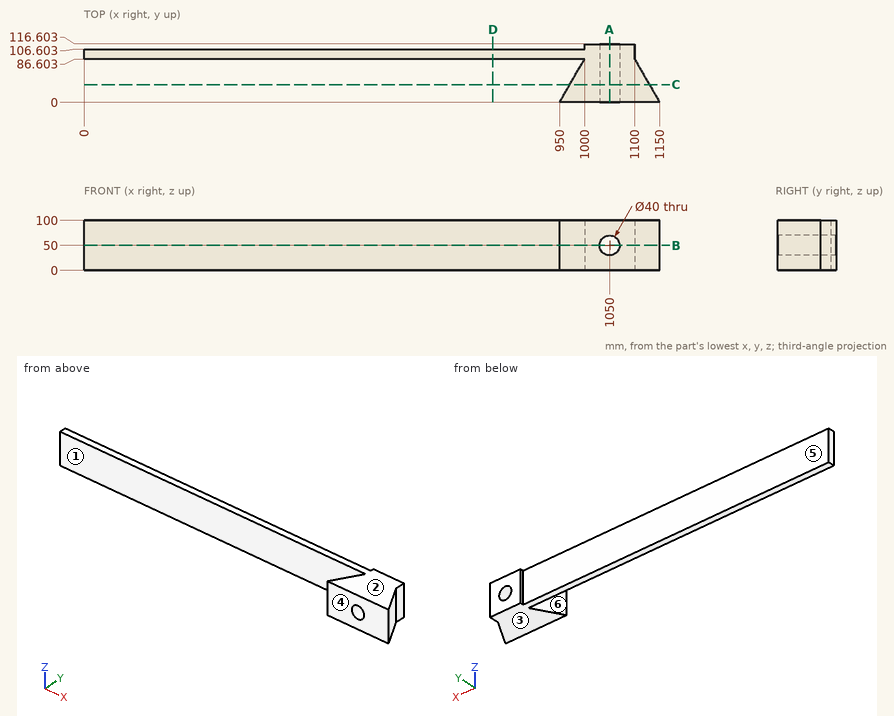
Could you check a few things on this drawing? It's one solid part, dimensions in mm from its lowest x, y, z. A direction names the side the tool comes from. Give positions to 0.01 mm unless a question says otherwise; leave off trailing zeros. Order: outer loops, then holes, each group sorted by start corner. A loop starts at its lowest first (then second) coordinate and runs counter-clockwise, first axis right, second up. Notation, with made-up numbers: (30, 64) - (40, 64) arc R19 cw to (40, 100) - close; hole circle Ø10 at (75.5, 69). An arc over 180 degrees is marked (long way). One line per item, written item: value. Start each with the question number.
1. Imagine slicing it at C-C on y = 35.5. List the corners of the cut face in (x, z) for me.
2. Imagine slicing it at D-D on x = 817. List the corners of the cut face in (y, z) for me.
3. For the marked faces 4, 5 and 6, which set-ups out of +Z, -Z, +X, -X, +Y, -Y let a thin tool reach every point of the face, with its end or its side?
4. Imagine slicing it at B-B on z = 50. List the corners of the cut face in (x, y) for me, plus the area to 3 significant figures.
5. For P1, Ø10, axis at x = 925, z = 40.5, coming from the +Y side; P2, Ø15, axis at y = 100, z = 66, coming from the +X side; P3, Ø8, axis at y = 25, z = 11, coming from the +X side (1 decimal), each with a flat end and sliding along its axis, tell me the tip position at first contact or that it passes through.
6. If I drill on probe 1 along Z at (x, y) = (1050, 31); probe 2 along Y at (x, z) = (817.5, 27); probe 3 along X at (y, z) = (82.5, 53) (1 decimal), over which ranges is the centre line in solid material (lowest first)?
7. Imagine slicing it at A-A on x = 1050. List the corners of the cut face in (y, z) for me.
8. Thinking about a two-plate mould opening in Z: for the marked faces 1, 2 and 3, which applies, +Z half, -Z half, draft (parallel to the pull), parting line (faces both ways), or undercut?
Values:
1. outline: (970.5, 0) - (1129.5, 0) - (1129.5, 100) - (970.5, 100) - close; hole circle Ø40 at (1050, 50)
2. outline: (86.6, 0) - (106.6, 0) - (106.6, 100) - (86.6, 100) - close
3. face 4: +Z, -Z, +X, -X, -Y
3. face 5: +Z, -Z, -X, +Y
3. face 6: +Z, -Z, -X
4. outline: (0, 86.6) - (1000, 86.6) - (950, 0) - (1030, 0) - (1030, 116.6) - (1000, 116.6) - (1000, 106.6) - (0, 106.6) - close; (1070, 0) - (1150, 0) - (1100, 86.6) - (1100, 116.6) - (1070, 116.6) - close
4. area: 31,300 mm²
5. P1: y = 106.6
5. P2: x = 1100
5. P3: x = 1137.9
6. probe 1: 0 to 30, 70 to 100
6. probe 2: 86.6 to 106.6
6. probe 3: 997.6 to 1030.2, 1069.8 to 1102.4
7. outline: (0, 0) - (116.6, 0) - (116.6, 30) - (0, 30) - close; (0, 70) - (116.6, 70) - (116.6, 100) - (0, 100) - close
8. face 1: draft
8. face 2: +Z half
8. face 3: -Z half
